```python
from build123d import *

# Parameters (mm, degrees)
F0_W           = 139.7
F0_H           = 139.7
F1_DEPTH       = 12.7
F2_R           = 18.25625
F2_R_2         = 16.1925
F3_DEPTH       = 9.525
F4_DEPTH       = 25.4
F7_D           = 6.35
F7_DEPTH       = 19.05
F7_TIP         = 1.9077324654
F7_ON_F6_D     = 6.35
F7_ON_F6_DEPTH = 19.05
F7_ON_F6_TIP   = 1.9077324654


with BuildPart() as f1:
    # F0 (on Top) → F1 (new body)
    with BuildSketch(Plane.XY):
        with Locations((7.4876705185, 11.5616054587)):
            Rectangle(F0_W, F0_H)
    extrude(amount=F1_DEPTH)

    # F2 (on face) → F3 (cut)
    with BuildSketch(Plane.XY.offset(12.7)):
        with Locations((7.4876705185, 11.5616054587)):
            Circle(F2_R)
        with Locations((7.4876705185, 11.5616054587)):
            Circle(F2_R_2, mode=Mode.SUBTRACT)
    extrude(amount=-F3_DEPTH, mode=Mode.SUBTRACT)

    # F4 (cut): a face of the model
    f4_faces = [f1.faces().sort_by_distance(p)[0] for p in [
        (7.4876705185, 11.5616054587, 12.7),
    ]]
    extrude(f4_faces, amount=-F4_DEPTH, mode=Mode.SUBTRACT)

    # F7
    with Locations(Plane.XZ.offset(58.2883945413)):
        with Locations((-56.0123294815, 6.35), (70.9876705185, 6.35)):
            Hole(F7_D / 2, depth=F7_DEPTH)
            with Locations((0, 0, -(F7_DEPTH + F7_TIP / 2))):  # 118° drill point
                Cone(0, F7_D / 2, F7_TIP, mode=Mode.SUBTRACT)

    # F7 on F6
    with Locations(Plane(origin=(0, 81.4116054587, 0), x_dir=(-1, 0, 0), z_dir=(0, 1, 0))):
        with Locations((-70.9876705185, 6.35), (56.0123294815, 6.35)):
            Hole(F7_ON_F6_D / 2, depth=F7_ON_F6_DEPTH)
            with Locations((0, 0, -(F7_ON_F6_DEPTH + F7_ON_F6_TIP / 2))):  # 118° drill point
                Cone(0, F7_ON_F6_D / 2, F7_ON_F6_TIP, mode=Mode.SUBTRACT)


solid = f1.part
```
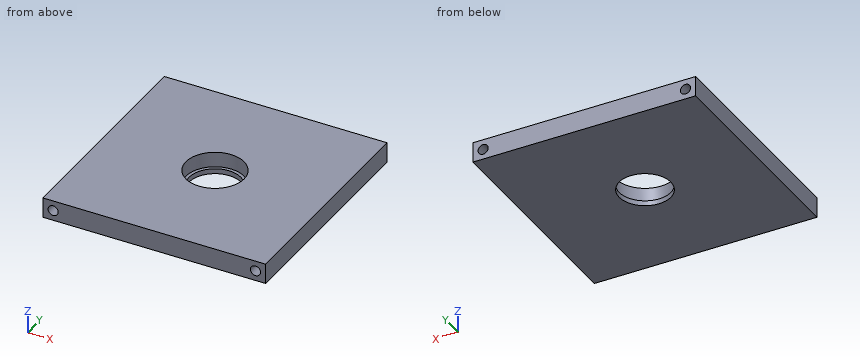
Input: part model. Units: mm. Frame: model coordinates. Coordinates: 2 decimals unless noted, no trailing zeros. Write each loop counter-clockwise with the first axis right and the second up, starting at its lowest first coordinate (ties: lowest second). Pieces come first, ordered by that corner, then holes.
1) Material intervals for line 1 along X through (y, z) = (-48.5, 6.35); line 2 along Y through (x, z) = (7.5, 5); line 3 along X through (y, z) = (7, 9.25), sorted ascending.
2) Section A-A on y = 25. Output: boundary loops of the cut face in (x, z) (3 decimals).
3) Pin query (flat end, axial travel): pin 1 Ø11 at (x, y) = (0, 3) entering from +Z (3 decimals); pin 2 Ø4 at (x, z) = (-56.01, 6.35) entering from +Y. Return the tip coordinate at first contact, or that it passes through.
4) Section B-B on y = -47. Output: boundary loops of the cut face in (x, z) (3 decimals).
Check result:
1. line 1: x = -62.36 to -59.19, -52.84 to 67.81, 74.16 to 77.34
1. line 2: y = -58.29 to -6.69, 29.82 to 81.41
1. line 3: x = -62.36 to -10.19, 25.16 to 77.34
2. outline: (-62.362, 0) - (-1.546, 0) - (-1.546, 3.175) - (-4.87, 3.175) - (-4.87, 12.7) - (-62.362, 12.7) - close; (16.521, 0) - (77.338, 0) - (77.338, 12.7) - (19.845, 12.7) - (19.845, 3.175) - (16.521, 3.175) - close
3. pin 1: stops at z = 3.175
3. pin 2: stops at y = 61.66
4. outline: (-62.362, 0) - (77.338, 0) - (77.338, 12.7) - (-62.362, 12.7) - close; hole circle Ø6.35 at (-56.012, 6.35); hole circle Ø6.35 at (70.988, 6.35)
